Model file for the job. Use its own axes, mm. Face numbers are marked on the shaded views. Give positions to 0.01 mm unless a question says otherwise; leave off trailing zeros. Order: outer loops, then holes, each group sorted by start corner. A loop starts at its lowest first (then second) coordinate and runs counter-clockwise, first axis right, second up. Notation, with made-up numbers: M -19.75,55 L 24.25,55 A30 ccw 24.25,86 Z; hole C -23.5,-33 d4. An arc over 180 degrees is marked long. Return JSON: item names as keys, results as strings. Group by question number.
1. Slice it at B-B on x = -9.5. List the corners of the cut face in (y, z).
2. Two-plate mould, pull along X, no slides. Class the marked faces 1, 2, 3 and 4: released by +X, released by -X, zero draft, split by the parting line, or undercut.
3. Slice it at A-A on y = 8.75. Give the number of separate pieces and of enclosed holes in the cut face, then the cut area to 3 significant figures.
4. Pin check, flat tips, straight feed: pin 1 (2 mm diameter, centred on x = 36, y = 5.5, fed in from +Z); pin 2 (5.5 mm diameter, centred on x = 36.12, y = 5, fed in from -Z). Stop position of each tip, or through.
5. Slice it at D-D on x = 43.5. List the corners of the cut face in (y, z), then the cut area to 3 significant figures.
6. Wall check: probe 1 along Z at (x, y) = (12, 4.25); probe 2 along Z at (x, y) = (42.5, 6); probe 3 along X at (y, z) = (1.25, 11.5). Give the ranges that are in metal, low to high. Write a range as [from, to].
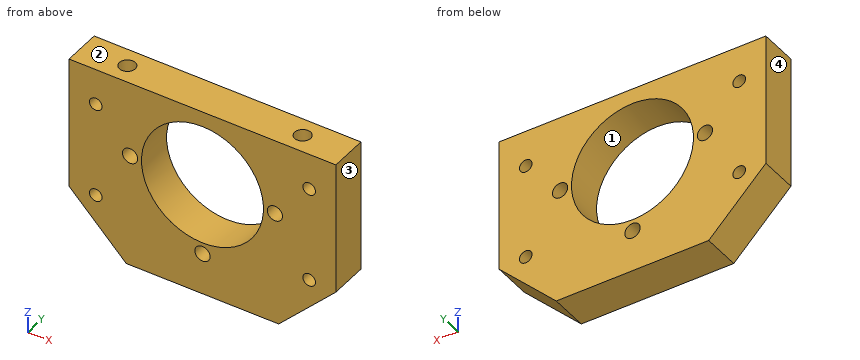
from build123d import *

# Parameters (mm, degrees)
SKETCH_1_W          = 70
SKETCH_1_H          = 50
SKETCH_1_R          = 16
EXTRUDE_1_DEPTH     = 10
CHAMFER_1_SIZE      = 15
SKETCH_4_R          = 2
CUT_EXTRUDE_3_DEPTH = 10
SKETCH_7_R          = 1.65
CUT_EXTRUDE_5_DEPTH = 10
SKETCH_8_R          = 2.1
CUT_EXTRUDE_6_DEPTH = 15


with BuildPart() as part:
    # Эскиз1 → Бобышка-Вытянуть1 (new body)
    with BuildSketch(Plane(origin=(0, 0, 0), x_dir=(1, 0, 0), z_dir=(0, 1, 0))):
        with Locations((13.122832672, -1.243812166)):
            Rectangle(SKETCH_1_W, SKETCH_1_H)
        with Locations(Location((13.122832672, -6.243812166, 0), (0, 0, 270))):
            Circle(SKETCH_1_R, mode=Mode.SUBTRACT)
    extrude(amount=EXTRUDE_1_DEPTH)

    # Фаска1
    chamfer_1_edges = [part.edges().sort_by_distance(p)[0] for p in [
        (-21.877167328, 5, -23.756187834),
        (48.122832672, 5, -23.756187834),
    ]]
    chamfer(chamfer_1_edges, length=CHAMFER_1_SIZE)

    # Эскиз4 → Вырез-Вытянуть3 (cut)
    with BuildSketch(Plane(origin=(0, 10, 0), x_dir=(1, 0, 0), z_dir=(0, 1, 0))):
        with Locations(Location((32.122832672, -6.243812166, 0), (0, 0, 270))):
            Circle(SKETCH_4_R)
        with Locations(Location((13.122832672, 12.756187834, 0), (0, 0, 270))):
            Circle(SKETCH_4_R)
        with Locations(Location((-5.877167328, -6.243812166, 0), (0, 0, 270))):
            Circle(SKETCH_4_R)
    extrude(amount=-CUT_EXTRUDE_3_DEPTH, mode=Mode.SUBTRACT)

    # Эскиз7 → Вырез-Вытянуть5 (cut)
    with BuildSketch(Plane(origin=(0, 10, 0), x_dir=(1, 0, 0), z_dir=(0, 1, 0))):
        with Locations(Location((41.122832672, 8.281187834, 0), (0, 0, 270))):
            Circle(SKETCH_7_R)
        with Locations(Location((41.122832672, -16.718812166, 0), (0, 0, 270))):
            Circle(SKETCH_7_R)
        with Locations(Location((-14.877167328, 8.281187834, 0), (0, 0, 270))):
            Circle(SKETCH_7_R)
        with Locations(Location((-14.877167328, -16.718812166, 0), (0, 0, 270))):
            Circle(SKETCH_7_R)
    extrude(amount=-CUT_EXTRUDE_5_DEPTH, mode=Mode.SUBTRACT)

    # Эскиз8 → Вырез-Вытянуть6 (cut)
    with BuildSketch(Plane.XY.offset(26.243812166)):
        with Locations((-9.877167328, 5)):
            Circle(SKETCH_8_R)
        with Locations((36.122832672, 5)):
            Circle(SKETCH_8_R)
    extrude(amount=-CUT_EXTRUDE_6_DEPTH, mode=Mode.SUBTRACT)


solid = part.part
Result:
{
 "1": {"outline": "M 0,-21.13 L 10,-21.13 L 10,26.24 L 7.07,26.24 L 7.07,11.24 L 2.93,11.24 L 2.93,26.24 L 0,26.24 Z"},
 "2": {"face 1": "undercut", "face 2": "zero draft", "face 3": "released by +X", "face 4": "released by -X"},
 "3": {"separate pieces": "1", "enclosed holes": "8", "area": "2,400 mm2"},
 "4": {"pin 1": "stops at z = 11.24", "pin 2": "stops at z = -23.51"},
 "5": {"outline": "M 0,-13.38 L 10,-13.38 L 10,26.24 L 0,26.24 Z", "area": "396 mm2"},
 "6": {"probe 1": "z = [-23.76, -14.41], [-11.1, -9.72], [22.2, 26.24]", "probe 2": "z = [-14.38, -9.19], [-7.37, 15.81], [17.63, 26.24]", "probe 3": "x = [-21.88, -1.99], [28.23, 48.12]"}
}
